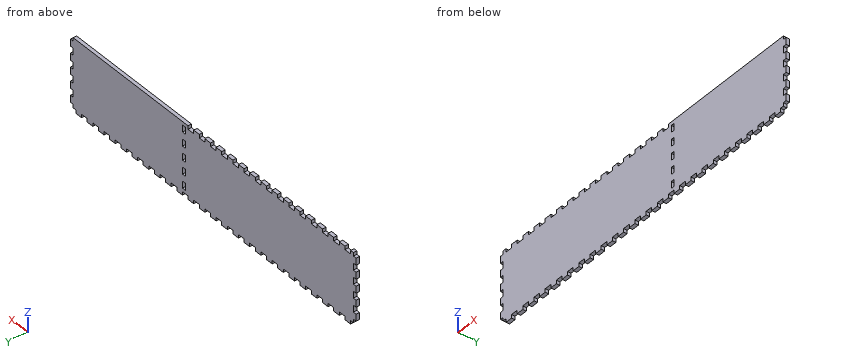
from build123d import *

# Parameters (mm, degrees)
SKETCH088_W             = 500
SKETCH088_H             = 100
PAD047_DEPTH            = 5
SKETCH089_W             = 10
SKETCH089_H             = 5
PAD048_DEPTH            = 5
LINEARPATTERN046_COUNT  = 25
LINEARPATTERN046_PITCH  = 20
SKETCH090_W             = 10
SKETCH090_H             = 5
PAD049_DEPTH            = 5
LINEARPATTERN047_COUNT  = 5
LINEARPATTERN047_PITCH  = 20
SKETCH091_W             = 10
SKETCH091_H             = 5
PAD050_DEPTH            = 5
LINEARPATTERN048_COUNT  = 5
LINEARPATTERN048_PITCH  = 20
SKETCH119_W             = 5
SKETCH119_H             = 10
POCKET029_DEPTH         = 5
LINEARPATTERN071_COUNT  = 5
LINEARPATTERN071_PITCH  = 20
SKETCH130_W             = 10
SKETCH130_H             = 5
POCKET039_DEPTH         = 5
LINEARPATTERN082_COUNT  = 15
LINEARPATTERN082_PITCH  = 20
BODY035_PLACEMENT_ANGLE = 90


with BuildPart() as part:
    # Sketch088 → Pad047 (new body)
    with BuildSketch(Plane.XY):
        Rectangle(SKETCH088_W, SKETCH088_H)
    extrude(amount=PAD047_DEPTH)

    # Sketch089 (on DatumPlane) → Pad048 (join)
    with BuildSketch(Plane.XZ.offset(50)):
        with Locations((-240, 2.5)):
            Rectangle(SKETCH089_W, SKETCH089_H)
    pad048 = extrude(amount=PAD048_DEPTH)

    # LinearPattern046: Pad048 ×25
    with Locations(*[(i * LINEARPATTERN046_PITCH, 0, 0) for i in range(1, LINEARPATTERN046_COUNT)]):
        add(pad048)

    # Sketch090 (on DatumPlane) → Pad049 (join)
    with BuildSketch(Plane.YZ.offset(250)):
        with Locations((-40, 2.5)):
            Rectangle(SKETCH090_W, SKETCH090_H)
    pad049 = extrude(amount=PAD049_DEPTH)

    # LinearPattern047: Pad049 ×5
    with Locations(*[(0, i * LINEARPATTERN047_PITCH, 0) for i in range(1, LINEARPATTERN047_COUNT)]):
        add(pad049)

    # Sketch091 (on DatumPlane) → Pad050 (join)
    with BuildSketch(Plane(origin=(-250, 0, 0), x_dir=(0, -1, 0), z_dir=(-1, 0, 0))):
        with Locations((-40, 2.5)):
            Rectangle(SKETCH091_W, SKETCH091_H)
    pad050 = extrude(amount=PAD050_DEPTH)

    # LinearPattern048: Pad050 ×5
    with Locations(*[(0, -i * LINEARPATTERN048_PITCH, 0) for i in range(1, LINEARPATTERN048_COUNT)]):
        add(pad050)

    # Sketch119 (on DatumPlane) → Pocket029 (cut)
    with BuildSketch(Plane(origin=(0, 0, 0), x_dir=(-1, 0, 0), z_dir=(0, 0, -1))):
        with Locations((-52.5, 40)):
            Rectangle(SKETCH119_W, SKETCH119_H)
    pocket029 = extrude(amount=-POCKET029_DEPTH, mode=Mode.SUBTRACT)

    # LinearPattern071: Pocket029 ×5
    with Locations(*[(0, -i * LINEARPATTERN071_PITCH, 0) for i in range(1, LINEARPATTERN071_COUNT)]):
        add(pocket029, mode=Mode.SUBTRACT)

    # Sketch130 (on DatumPlane) → Pocket039 (cut)
    with BuildSketch(Plane(origin=(0, 50, 0), x_dir=(-1, 0, 0), z_dir=(0, 1, 0))):
        with Locations((240, 2.5)):
            Rectangle(SKETCH130_W, SKETCH130_H)
    pocket039 = extrude(amount=-POCKET039_DEPTH, mode=Mode.SUBTRACT)

    # LinearPattern082: Pocket039 ×15
    with Locations(*[(i * LINEARPATTERN082_PITCH, 0, 0) for i in range(1, LINEARPATTERN082_COUNT)]):
        add(pocket039, mode=Mode.SUBTRACT)


with BuildPart() as part_1:
    # Body035 placement: moved
    add(part.part.moved(Location((0, -45, 55))).rotate(Axis((0, -45, 55), (1, 0, 0)), BODY035_PLACEMENT_ANGLE))


solid = part_1.part
Verification items for the finished model (mm, model axes). Round coordinates to 2 decimals unless told otherwise and drop trailing zeros. Put each result on its own line as item: value.
1) Material ranges on line 1 (X direction, y = -46.85, z = 17); line 2 (X direction, y = -47.4, z = 48); line 3 (Z direction, x = -19, y = -48.1), recorded low to high.
Final values:
line 1: x = -255 to 50, 55 to 255
line 2: x = -250 to 250
line 3: z = 0 to 100
2) Depth check by flat-ended pin: pin 1 (2.5 mm diameter, centred on y = -48.5, z = 103.5, fed in from -X); pin 2 (2.5 mm diameter, centred on y = -46.5, z = 3.5, fed in from -X); pin 3 (1.5 mm diameter, centred on x = -253.5, y = -46.5, fed in from +Z). Enter the tip coordinate at first touch or a pass-through.
Final values:
pin 1: stops at x = -250
pin 2: stops at x = -245
pin 3: stops at z = 100
3) Section check A-A (y = -46.3). Give the number of separate pieces and of enclosed holes in the cut face, then the cut area to 4 significant figures.
Final values:
separate pieces: 1
enclosed holes: 5
area: 50,750 mm^2
